Could you check a few things on this model? Use its own coordinates, in mm. Face numbers are marked on the shaded views. A direction names the side the tool comes from. Coordinates: 2 decimals unless noted, no trailing zeros. Loops run counter-clockwise (first coordinate to the right, second up) from the corner with the lowest first, then second, coordinate; pieces in that order, holes last.
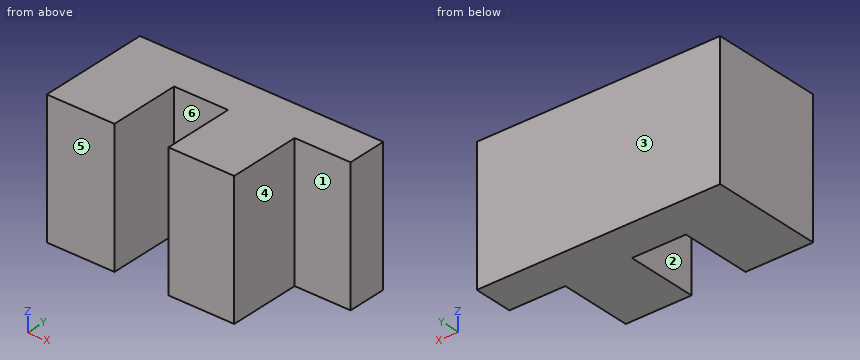
from build123d import *

# Parameters (mm, degrees)
F0_W     = 108.822718
F0_H     = 59.676976
F1_DEPTH = 50
F2_W     = 32.45962
F2_H     = 59.676976
F3_DEPTH = 25
F4_W     = 24.134072
F4_H     = 32.020826
F5_DEPTH = 25
F6_DEPTH = 60


with BuildPart() as f1:
    # F0 (on Front) → F1 (new body)
    with BuildSketch(Plane.XZ):
        Rectangle(F0_W, F0_H)
    extrude(amount=-F1_DEPTH)

    # F2 (on face) → F3 (cut)
    with BuildSketch(Plane.YZ.offset(54.411359)):
        with Locations((16.22981, 0)):
            Rectangle(F2_W, F2_H)
    extrude(amount=-F3_DEPTH, mode=Mode.SUBTRACT)

    # F4 (on face) → F5 (cut)
    with BuildSketch(Plane.XY.offset(29.838488)):
        with Locations((-12.067036, 16.010413)):
            Rectangle(F4_W, F4_H)
    extrude(amount=F5_DEPTH, mode=Mode.SUBTRACT)

    # F4 (on face) → F6 (cut)
    with BuildSketch(Plane.XY.offset(29.838488)):
        with Locations((-12.067036, 16.010413)):
            Rectangle(F4_W, F4_H)
    extrude(amount=-F6_DEPTH, mode=Mode.SUBTRACT)


solid = f1.part
(1) Imagine slicing it at A-A, the plane y = 10.5. Write out the boundary of the cut face in (x, z).
Answers:
outline: (-54.41, -29.84) - (-24.13, -29.84) - (-24.13, 29.84) - (-54.41, 29.84) - close; (0, -29.84) - (29.41, -29.84) - (29.41, 29.84) - (0, 29.84) - close
(2) Which directions (+Z, -Z, +X, -X, +Y, -Y) give clear straight access to the entire face, cutting with the end or side of a thin tool? Please do the marked faces 1, 2 and 3.
Answers:
face 1: +Z, -Z, +X, -Y
face 2: +Z, -Z, -Y
face 3: +Z, -Z, +X, -X, +Y
(3) Imagine slicing it at D-D, the plane x = 35.5. Write out the boundary of the cut face in (y, z), and give its area (3 significant figures).
Answers:
outline: (32.46, -29.84) - (50, -29.84) - (50, 29.84) - (32.46, 29.84) - close
area: 1,050 mm2
(4) We'd pull the mould along X, two halves only. Please class the marked faces 4, 5 and 6: +X half, -X half, draft (parallel to the pull), parting line (faces both ways), or undercut.
Answers:
face 4: +X half
face 5: draft
face 6: undercut
(5) Imagine slicing it at C-C, the plane x = -18. Write out the boundary of the cut face in (y, z), and give its area (3 significant figures).
Answers:
outline: (32.02, -29.84) - (50, -29.84) - (50, 29.84) - (32.02, 29.84) - close
area: 1,070 mm2
(6) I need wall thicknesses on probe 1 along X at (y, z) = (19.5, 27.5); probe 2 along Y at (x, z) = (-17.5, 7); probe 3 along Y at (x, z) = (39.5, 13.5). Which ranges of each line are inside material? Lowest first, please.
Answers:
probe 1: x = -54.41 to -24.13, 0 to 29.41
probe 2: y = 32.02 to 50
probe 3: y = 32.46 to 50
(7) Imagine slicing it at B-B, the plane z = 12.5. Write out the boundary of the cut face in (x, y).
Answers:
outline: (-54.41, 0) - (-24.13, 0) - (-24.13, 32.02) - (0, 32.02) - (0, 0) - (29.41, 0) - (29.41, 32.46) - (54.41, 32.46) - (54.41, 50) - (-54.41, 50) - close
(8) For pin 1 (9.5 mm diameter, centred on y = 11.5, z = -11, fed in from +X); pin 2 (12.5 mm diameter, centred on x = 47.5, z = 11, fed in from -Y), each with a flat end and sliding along its axis, tell me the tip position at first contact or that it passes through.
Answers:
pin 1: stops at x = 29.41
pin 2: stops at y = 32.46
